Here's the drawing with two shaded views (mm, measured from the low corner). I have some questions. A direction names the side the tool comes from. Round coordinates to 2 decimals unless told otherwise and drop trailing zeros. Loops run counter-clockwise (first coordinate to the right, second up) from the corner with the lowest first, then second, coordinate; pieces in that order, holes last.
(1) If I drill on line 1 along X through (y, z) = (4.5, 31.75); line 2 along X through (y, z) = (0.5, 41.5) (3 decimals), over which ranges is the centre line in solid material (lowest first)?
(2) I want a section at D-D on z = 44. Write out the boundary of the cut face in (x, y) (3 decimals), plus the area to 3 significant figures.
(3) Which directions (+Z, -Z, +X, -X, +Y, -Y) give clear straight access to the entire face, cutting with the end or side of a thin tool? Please do the marked faces 1, 2, 3, 4 and 5.
(4) I want a section at A-A on x = 31.75. Write out the boundary of the cut face in (y, z).
(5) I want a section at B-B on z = 31.75. Write out the boundary of the cut face in (x, y), plus the area to 3 significant figures.
(6) Will these pins go through, and if not, where does the flat tip stop? pin 1 Ø2.5 at (x, y) = (51.5, 3) entering from +Z (3 decimals); pin 2 Ø2.5 at (y, z) = (3.5, 11) entering from -X (3 decimals); pin 3 Ø1.5 at (y, z) = (1.5, 55.5) entering from +X (3 decimals).
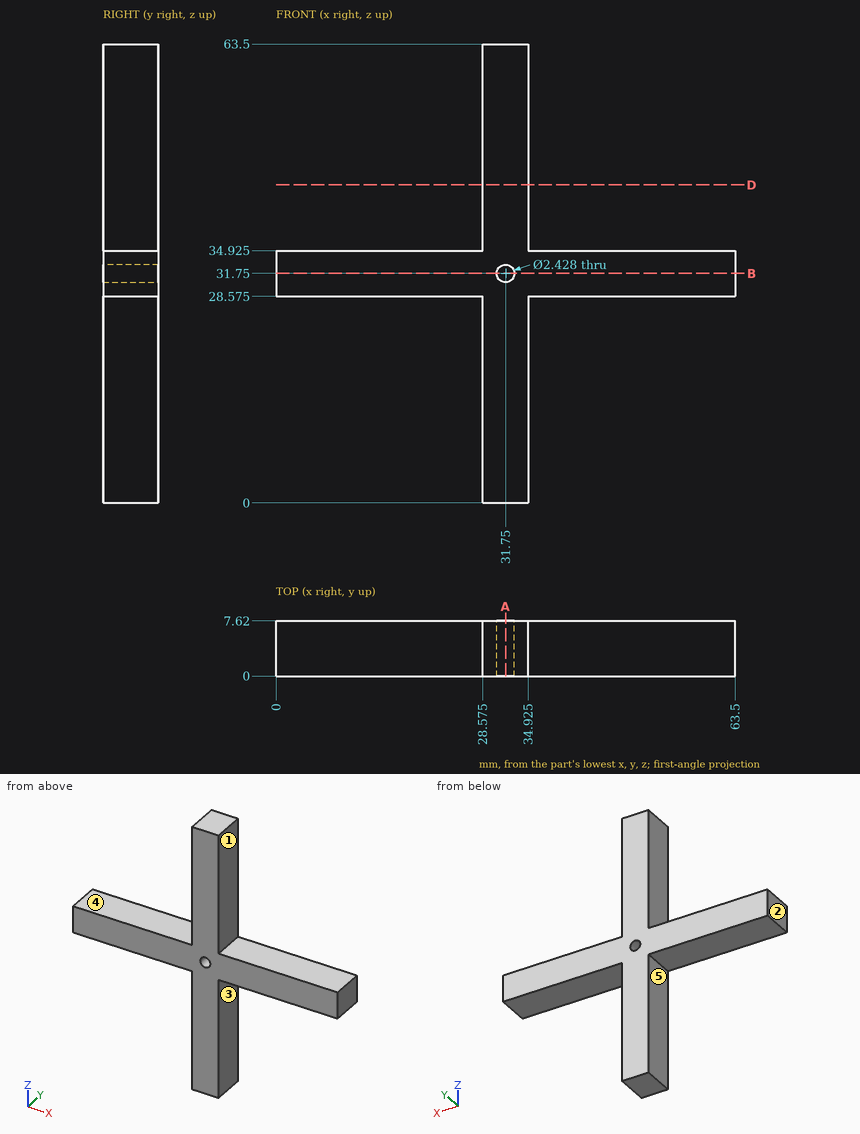
Filled sheet:
1. line 1: x = 0 to 30.54, 32.96 to 63.5
1. line 2: x = 28.575 to 34.925
2. outline: (28.575, 0) - (34.925, 0) - (34.925, 7.62) - (28.575, 7.62) - close
2. area: 48.4 mm2
3. face 1: +Z, +X, +Y, -Y
3. face 2: +Z, -Z, -X, +Y, -Y
3. face 3: -Z, +X, +Y, -Y
3. face 4: +Z, -X, +Y, -Y
3. face 5: -Z, -X, +Y, -Y
4. outline: (0, 0) - (7.62, 0) - (7.62, 30.54) - (0, 30.54) - close; (0, 32.96) - (7.62, 32.96) - (7.62, 63.5) - (0, 63.5) - close
5. outline: (0, 0) - (30.54, 0) - (30.54, 7.62) - (0, 7.62) - close; (32.96, 0) - (63.5, 0) - (63.5, 7.62) - (32.96, 7.62) - close
5. area: 465 mm2
6. pin 1: stops at z = 34.925
6. pin 2: stops at x = 28.575
6. pin 3: stops at x = 34.925
